Part print with two shaded views. Sizes in mm from the minimum x, y, z corner. Round coordinates to 2 decimals unless told otherwise and drop trailing zeros. Loops run counter-clockwise (first coordinate to the right, second up) from the corner with the lowest first, then second, coordinate; pieces in that order, holes last.
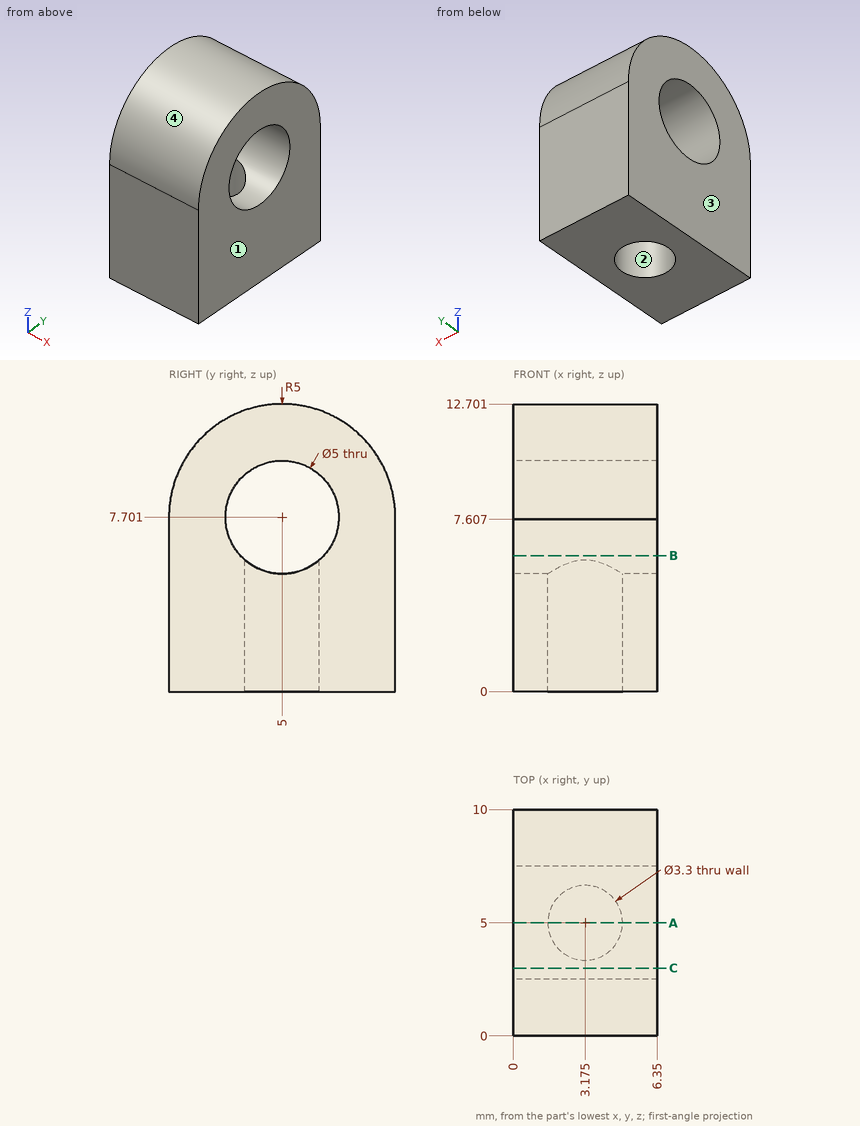
Item 1: Wall check: L1, parallel to Y at x = 1.75, z = 4.75 (1 decimal); L2, parallel to Z at x = 3.75, y = 3 (1 decimal); L3, parallel to Z at x = 5, y = 5.75 (1 decimal). Give the ranges that are in metal, low to high.
Verdict:
L1: y = 0 to 4.2, 5.8 to 10
L2: z = 0 to 6.2, 9.2 to 12.3
L3: z = 0 to 5.3, 10.1 to 12.6
Item 2: Cut at A-A (y = 5). State how many separate pieces and enclosed holes the cut face has.
Verdict:
separate pieces: 3
enclosed holes: 0
Item 3: Cut at B-B (z = 6). List the corners of the cut face in (x, y).
Verdict:
outline: (0, 0) - (6.35, 0) - (6.35, 3.17) - (0, 3.17) - close; (0, 6.83) - (6.35, 6.83) - (6.35, 10) - (0, 10) - close
Item 4: Flat gauge pins, fed straight in: P1, Ø1.5, axis at x = 5, y = 7.5, coming from the +Z side (1 decimal); P2, Ø3, axis at x = 3.175, y = 5, coming from the -Z side; P3, Ø4.5, axis at y = 5, z = 7.7, coming from the +X side. Where does each tip first touch, or does it go through?
Verdict:
P1: stops at z = 12.4
P2: stops at z = 9.7
P3: passes through
Item 5: Mould opens along X. For the marked faces 1, 2, 3 and 4 say: released by +X, released by -X, zero draft, split by the parting line, or undercut.
Verdict:
face 1: released by +X
face 2: undercut
face 3: released by -X
face 4: zero draft
Item 6: Cut at C-C (y = 3). List the corners of the cut face in (x, z).
Verdict:
outline: (0, 0) - (6.35, 0) - (6.35, 6.2) - (0, 6.2) - close; (0, 9.2) - (6.35, 9.2) - (6.35, 12.28) - (0, 12.28) - close
